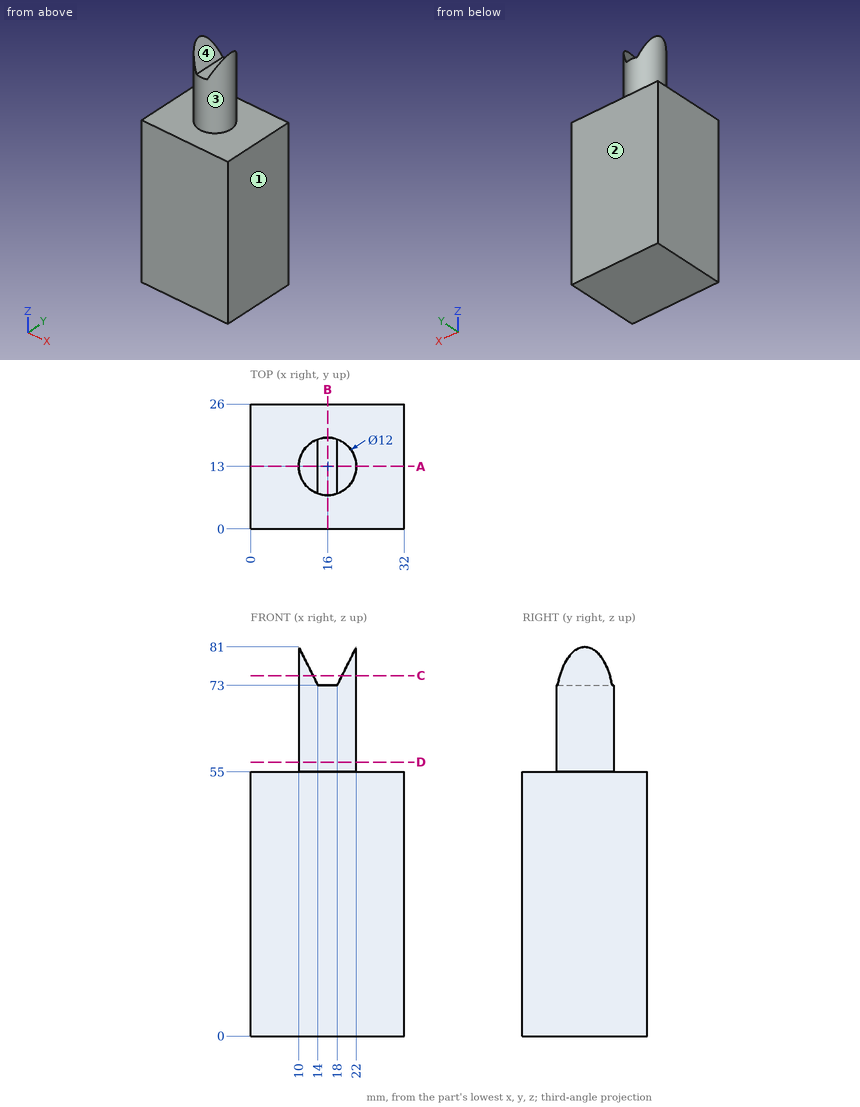
Part print with two shaded views. Sizes in mm from the minimum x, y, z corner. Give positions to 0.01 mm unless a question says otherwise; leave off trailing zeros. Order: outer loops, then holes, each group sorted by start corner. A loop starts at its lowest first (then second) coordinate and runs counter-clockwise, first axis right, second up.
1) Saw through at D-D, the plane z = 57. Write the cut outline in (x, y), then the cut area to 3 significant figures.
2) Pin check, flat tips, straight feed: pin 1 (2 mm diameter, centred on x = 22.5, z = 65, fed in from +Y); pin 2 (8 mm diameter, centred on y = 12, z = 33, fed in from -X); pin 3 (1.2 mm diameter, centred on x = 15, y = 12.5, fed in from +Z). Stop position of each tip, or through.
3) Saw through at A-A, the plane y = 13. Write the cut outline in (x, z).
4) Saw through at C-C, the plane z = 75. Write the cut outline in (x, y).
5) Saw through at B-B, the plane x = 16. Write the cut outline in (y, z), then the cut area to 3 significant figures.
6) Mould opens along X. For the marked faces 1, 2, 3 and 4 say: +X half, -X half, draft (parallel to the pull), parting line (faces both ways), or undercut.
7) Wall check: probe 1 along Z at (x, y) = (9.5, 9.5); probe 2 along Z at (x, y) = (17, 8); probe 3 along Y at (x, z) = (17.5, 72.5). Give the ranges that are in metal, low to high.
Computed:
1. outline: circle Ø12 at (16, 13)
1. area: 113 mm2
2. pin 1: stops at y = 15.4
2. pin 2: stops at x = 0
2. pin 3: stops at z = 73
3. outline: (0, 0) - (32, 0) - (32, 55) - (22, 55) - (22, 81) - (18, 73) - (14, 73) - (10, 81) - (10, 55) - (0, 55) - close
4. outline: (13, 7.8) - (13, 18.2) arc R6 ccw to start; (19, 7.8) arc R6 ccw to (19, 18.2) - close
5. outline: (0, 0) - (26, 0) - (26, 55) - (19, 55) - (19, 73) - (7, 73) - (7, 55) - (0, 55) - close
5. area: 1,650 mm2
6. face 1: +X half
6. face 2: draft
6. face 3: parting line
6. face 4: undercut
7. probe 1: z = 0 to 55
7. probe 2: z = 0 to 73
7. probe 3: y = 7.19 to 18.81
